Geometry: final body of the model. Coordinates: model frame, mm. A direction names the side the tool comes from. Round coordinates to 2 decimals unless told otherwise and drop trailing zeros. Loops run counter-clockwise (first coordinate to the right, second up) from the corner with the lowest first, then second, coordinate; pieces in that order, holes last. Notation, with made-up numbers: (-11, -13.75) - (20, -13.75) arc R33 cw to (20, 19.25) - close; hole circle Ø1 at (-1.5, 0.5). An arc over 180 degrees is marked (long way). Return JSON: item names as keys, results as strings. Group by question number.
1. Section C-C on z = 6.75. Return loops of the section in (x, y).
2. First-contact query: pin 1 Ø2.5 at (x, y) = (0, -12) entering from -Z; pin 2 Ø6 at (x, z) = (2.5, 9.5) entering from +Y; pin 3 Ø5 at (x, z) = (0, 8.5) entering from -Y. Flat tips, straight axial feed; report the tip coordinate or a pass-through.
3. Section B-B on x = 0. Return loops of the section in (y, z).
4. Material intervals for probe 1 along Y at (x, z) = (0, 0.05); probe 2 along X at (y, z) = (-11.25, 1.5); probe 3 along Y at (x, z) = (-1.5, 3.25), sorted ascending.
5. Section A-A on y = -12. Return loops of the section in (x, z).
6. Draft query along X for faces 1 (the face through (5, -8, 2)), 2 (the face through (1, -9.9, -2.5)), 3 (the face through (-2.15, -11.91, 0.04)). Return one class per face: +X half, -X half, draft (parallel to the pull), parting line (faces both ways), or undercut.
7. Set-up query: faces 4 (the face through (0, -3, 12.5)), 5 (the face through (-1.2, -14.1, 2.5)). Return all of +Z, -Z, +X, -X, +Y, -Y with unobstructed straight access to the full face (end or side cutting, diameter ignored); none if empty.
8. Section D-D on z = 2.25. Return loops of the section in (x, y).
from build123d import *

# Parameters (mm, degrees)
F0_W     = 10
F0_H     = 5
F1_DEPTH = 20
F2_W     = 5
F2_H     = 10
F3_DEPTH = 5
F4_R     = 2.15
F5_DEPTH = 12.5
F6_R     = 2.15
F7_DEPTH = 5.1


with BuildPart() as f1:
    # F0 (on Front) → F1 (new body)
    with BuildSketch(Plane.XZ):
        Rectangle(F0_W, F0_H)
    extrude(amount=F1_DEPTH)

    # F2 (on Right) → F3 (join, symmetric)
    with BuildSketch(Plane.YZ):
        with Locations((-2.5, 7.5)):
            Rectangle(F2_W, F2_H)
    extrude(amount=F3_DEPTH, both=True)

    # F4 (on Top) → F5 (cut, symmetric)
    with BuildSketch(Plane.XY):
        with Locations((0, -12)):
            Circle(F4_R)
    extrude(amount=F5_DEPTH, both=True, mode=Mode.SUBTRACT)

    # F6 (on Front) → F7 (cut)
    with BuildSketch(Plane.XZ):
        with Locations((0, 7.5)):
            Circle(F6_R)
    extrude(amount=F7_DEPTH, mode=Mode.SUBTRACT)


solid = f1.part
Taken from the geometry:
{
 "1": {"outline": "(-5, -5) - (-2.01, -5) - (-2.01, 0) - (-5, 0) - close; (2.01, -5) - (5, -5) - (5, 0) - (2.01, 0) - close"},
 "2": {"pin 1": "through", "pin 2": "y = 0", "pin 3": "y = -5"},
 "3": {"outline": "(-20, -2.5) - (-14.15, -2.5) - (-14.15, 2.5) - (-20, 2.5) - close; (-9.85, -2.5) - (0, -2.5) - (0, 5.35) - (-5, 5.35) - (-5, 2.5) - (-9.85, 2.5) - close; (-5, 9.65) - (0, 9.65) - (0, 12.5) - (-5, 12.5) - close"},
 "4": {"probe 1": "-20 to -14.15, -9.85 to 0", "probe 2": "-5 to -2.01, 2.01 to 5", "probe 3": "-5 to 0"},
 "5": {"outline": "(-5, -2.5) - (-2.15, -2.5) - (-2.15, 2.5) - (-5, 2.5) - close; (2.15, -2.5) - (5, -2.5) - (5, 2.5) - (2.15, 2.5) - close"},
 "6": {"face 1": "+X half", "face 2": "draft", "face 3": "undercut"},
 "7": {"face 4": "+Z, +X, -X, +Y, -Y", "face 5": "+Z, +X, -X, -Y"},
 "8": {"outline": "(-5, -20) - (5, -20) - (5, 0) - (-5, 0) - close; hole circle Ø4.3 at (0, -12)"}
}
